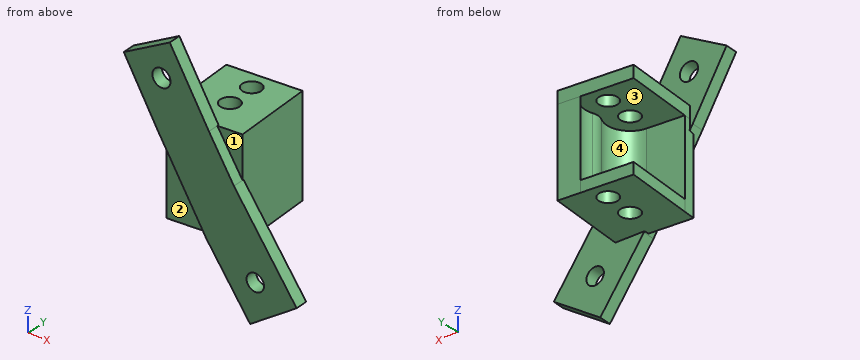
from build123d import *

# Parameters (mm, degrees)
BOSS_EXTRUDE1_DEPTH = 29.21
SKETCH2_R           = 3.175
SKETCH2_R_2         = 3.150896054
BOSS_EXTRUDE2_DEPTH = 4.064
BOSS_EXTRUDE3_START = -3.81
SKETCH3_R           = 3.150896054
SKETCH3_R_2         = 3.175
BOSS_EXTRUDE3_DEPTH = 3.81
SKETCH4_R           = 2.912114347
SKETCH4_R_2         = 3.035248441
BOSS_EXTRUDE4_DEPTH = 4.064


with BuildPart() as part:
    # Sketch1 → Boss-Extrude1 (new body)
    with BuildSketch(Plane.XY):
        with BuildLine():
            Line((-184.947787902, 216.023814704), (-197.134551999, 215.040325013))
            Line((-197.134551999, 215.040325013), (-196.807644057, 210.989494579))
            Line((-196.807644057, 210.989494579), (-172.630398999, 212.940633626))
            Line((-172.630398999, 212.940633626), (-174.867675228, 240.663504402))
            Line((-174.867675228, 240.663504402), (-182.112910704, 240.0788033))
            ThreePointArc((-182.112910704, 240.0788033), (-179.090453568, 236.146361834), (-179.097761142, 231.186594741))
            ThreePointArc((-179.097761142, 231.186594741), (-179.357825473, 229.166849047), (-178.803768808, 227.207250277))
            ThreePointArc((-178.803768808, 227.207250277), (-178.89422454, 219.977509591), (-184.947787902, 216.023814704))
        make_face()
    extrude(amount=-BOSS_EXTRUDE1_DEPTH)

    # Sketch2 → Boss-Extrude2 (add)
    with BuildSketch(Plane.XY):
        Polygon((-174.867675228, 240.663504402), (-172.630398999, 212.940633626), (-196.807644057, 210.989494579), (-199.044920286, 238.712365356), align=None)
        with Locations((-185.628460018, 223.67720197)):
            Circle(SKETCH2_R, mode=Mode.SUBTRACT)
        with Locations((-186.37244208, 233.67720197)):
            Circle(SKETCH2_R_2, mode=Mode.SUBTRACT)
    extrude(amount=BOSS_EXTRUDE2_DEPTH)

    # Sketch3 → Boss-Extrude3 (add)
    with BuildSketch(Plane(origin=(0, 0, -29.21), x_dir=(-1, 0, 0), z_dir=(0, 0, -1)).offset(BOSS_EXTRUDE3_START)):
        with BuildLine():
            Line((197.134551999, 215.040325013), (199.044920286, 238.712365356))
            Line((199.044920286, 238.712365356), (182.112910704, 240.0788033))
            ThreePointArc((182.112910704, 240.0788033), (179.090453568, 236.146361834), (179.097761142, 231.186594741))
            ThreePointArc((179.097761142, 231.186594741), (179.357825473, 229.166849047), (178.803768808, 227.207250277))
            ThreePointArc((178.803768808, 227.207250277), (178.89422454, 219.977509591), (184.947787902, 216.023814704))
            Line((184.947787902, 216.023814704), (197.134551999, 215.040325013))
        make_face()
        with Locations(Location((186.37244208, 233.67720197, 0), (0, 0, 180))):
            Circle(SKETCH3_R, mode=Mode.SUBTRACT)
        with Locations(Location((185.628460018, 223.67720197, 0), (0, 0, 180))):
            Circle(SKETCH3_R_2, mode=Mode.SUBTRACT)
    extrude(amount=BOSS_EXTRUDE3_DEPTH)

    # Sketch4 → Boss-Extrude4 (add)
    with BuildSketch(Plane(origin=(-3.401075391, 215.535251129, 6.555182159), x_dir=(0.9998756392437431, 0.015763128213975516, 0.0004794119583323757), z_dir=(-0.01577041682759283, 0.9994135267149824, 0.030395666997208134))):
        Polygon((-178.918526698, 35.997686208), (-164.828562801, 57.087586654), (-149.044849512, 46.542636431), (-169.257027987, 16.288986745), (-177.265593638, 2.391514831), (-189.802185869, -20.421476842), (-205.369032328, -11.866912445), (-194.539107817, 8.279817663), align=None)
        with Locations(Location((-162.788777802, 43.630522083, 0), (0, 0, 270))):
            Circle(SKETCH4_R, mode=Mode.SUBTRACT)
        with Locations(Location((-192.870314924, -8.404113006, 0), (0, 0, 270))):
            Circle(SKETCH4_R_2, mode=Mode.SUBTRACT)
    extrude(amount=-BOSS_EXTRUDE4_DEPTH)


solid = part.part
Build history of the part. All positions in model axes, mm. Face numbers are marked on the shaded views. Give positions to 0.01 mm unless a question says otherwise; leave off trailing zeros. Order: outer loops, then holes, each group sorted by start corner. A loop starts at its lowest first (then second) coordinate and runs counter-clockwise, first axis right, second up. Notation, with made-up numbers: M 67,43 L 89,43 A18 ccw 89,56 Z; hole C -36.75,14 d7. An arc over 180 degrees is marked long. Use one line per item in the form item = value.
1) Drop flat-ended pins along their axis: pin 1 (4 mm diameter, centred on y = 215.5, z = 8, fed in from -X); pin 2 (6 mm diameter, centred on x = -201, y = 236.5, fed in from +Z); pin 3 (3 mm diameter, centred on y = 229.5, z = -25.5, fed in from +X); pin 4 (8 mm diameter, centred on x = -200.5, y = 237, fed in from -Z). Give the stop position or say it passes through.
Calculated:
pin_1 = through
pin_2 = 4.06
pin_3 = -173.85
pin_4 = -29.21
2) Probe probe 1 along Z at (x, y) = (-197, 216.5); probe 2 along Y at (x, z) = (-203, 15); probe 3 along X at (y, z) = (225, -26). List the from-to ranges inside material, lowest first.
Calculated:
probe_1 = -29.21 to -25.4, 0 to 4.06
probe_2 = 208.06 to 212.13
probe_3 = -197.94 to -188.51, -182.74 to -173.6
3) Two-plate mould, pull along X, no slides. Class the marked faces 1, 2, 3 and 4: released by +X, released by -X, zero draft, split by the parting line, or undercut.
Calculated:
face_1 = released by +X
face_2 = undercut
face_3 = zero draft
face_4 = released by -X
4) Saw through at B-B (y = 235). Give the cut face in (x, z).
Calculated:
outline = M -198.75,-29.21 L -189.23,-29.21 L -189.23,-25.4 L -198.75,-25.4 Z; M -198.75,0 L -189.23,0 L -189.23,4.06 L -198.75,4.06 Z; M -183.51,-29.21 L -174.41,-29.21 L -174.41,4.06 L -183.51,4.06 L -183.51,0 L -178.8,0 L -178.8,-25.4 L -183.51,-25.4 Z
5) Saw through at C-C (z = -7). Give the cut face in (x, y).
Calculated:
outline = M -197.13,215.04 L -196.81,210.99 L -194.99,211.14 L -195,208.86 L -174.26,209.18 L -174.26,212.81 L -172.63,212.94 L -174.87,240.66 L -182.11,240.08 A7.69 cw -179.1,231.19 A5.08 ccw -178.8,227.21 A7.68 cw -184.95,216.02 Z
6) Saw through at A-A (z = 2.5). State how many separate pieces and enclosed holes the cut face has, plus the area to 3 significant figures.
Calculated:
separate_pieces = 1
enclosed_holes = 2
area = 677 mm2
7) Saw through at D-D (y = 229.5). Give the cut face in (x, z).
Calculated:
outline = M -198.3,-29.21 L -173.97,-29.21 L -173.97,4.06 L -198.3,4.06 L -198.3,0 L -179.37,0 L -179.37,-25.4 L -198.3,-25.4 Z
